from build123d import *

# Parameters (mm, degrees)
SKETCH1_W           = 650
SKETCH1_H           = 90
BOSS_EXTRUDE1_DEPTH = 90
SKETCH2_R           = 25
BOSS_EXTRUDE2_DEPTH = 35


with BuildPart() as part:
    # Sketch1 → Boss-Extrude1 (new body)
    with BuildSketch(Plane.XY):
        with Locations((325, 45)):
            Rectangle(SKETCH1_W, SKETCH1_H)
    extrude(amount=BOSS_EXTRUDE1_DEPTH)

    # Sketch2 → Boss-Extrude2 (add)
    with BuildSketch(Plane(origin=(0, 90, 0), x_dir=(1, 0, 0), z_dir=(0, 1, 0))):
        with Locations(Location((63.60842931, -47.01070439, 0), (0, 0, 90))):  # turned: the seam where the file's is
            Circle(SKETCH2_R)
        with Locations(Location((563.60842931, -47.01070439, 0), (0, 0, 90))):  # turned: the seam where the file's is
            Circle(SKETCH2_R)
    extrude(amount=BOSS_EXTRUDE2_DEPTH)


solid = part.part
Source: CAD feature listing. Evaluate the final solid. Frame: model axes, mm. Coordinates: 2 decimals unless noted, no trailing zeros. Loops run counter-clockwise (first coordinate to the right, second up) from the corner with the lowest first, then second, coordinate; pieces in that order, holes last. Notation, with made-up numbers: (65, 65.5) - (77, 65.5) arc R12 cw to (77, 79.5) - close; hole circle Ø1 at (44.5, -15.5). An arc over 180 degrees is marked (long way). One line per item, written item: value. Start each with the question number.
1. Mould query, pull axis X, two halves, no side actions, for faces 1 (the flat face through (650, 44, 44)), 2 (the cylindrical face through (85.8, 107.3, 35.5)), 3 (the cylindrical face through (538.82, 107.26, 50.27)), 4 (the flat face through (320, 46, 0)). Classes: pulls with the +X half, pulls with the -X half, needs draft (parallel to the pull), parting line crosses it, or undercut.
2. Contact query for a flat-ended pin moving along its axis: P1, Ø1.5, axis at y = 101.5, z = 33, coming from the +X side. Output: stop coordinate, or through.
3. Section B-B (x = 165). Return the cut outline in (y, z).
4. Section A-A (z = 51). Return the cut outline in (x, y), and give its area (3 significant figures).
5. Ray query, L1, parallel to Y at x = 585, z = 77.5. Return the intervals inside material, ascending.
Verdict:
1. face 1: pulls with the +X half
1. face 2: undercut
1. face 3: undercut
1. face 4: needs draft
2. P1: stops at x = 584.8
3. outline: (0, 0) - (90, 0) - (90, 90) - (0, 90) - close
4. outline: (0, 0) - (650, 0) - (650, 90) - (588.29, 90) - (588.29, 125) - (538.93, 125) - (538.93, 90) - (88.29, 90) - (88.29, 125) - (38.93, 125) - (38.93, 90) - (0, 90) - close
4. area: 62,000 mm2
5. L1: y = 0 to 90
